from build123d import *

# Parameters (mm, degrees)
SKETCH1_R           = 2.5
SKETCH1_R_2         = 3.5
SKETCH1_R_3         = 1.5
SKETCH1_W           = 3
SKETCH1_H           = 10
BOSS_EXTRUDE3_DEPTH = 3


with BuildPart() as part:
    # Sketch1 → Boss-Extrude3 (new body)
    with BuildSketch(Plane(origin=(0, 0, 0), x_dir=(1, 0, 0), z_dir=(0, 1, 0))):
        with BuildLine():
            Line((36.277091695, 79.255784564), (46.277091695, 79.255784564))
            Line((46.277091695, 79.255784564), (46.277091695, 76.347710002))
            Line((46.277091695, 76.347710002), (71.277091695, 76.347710002))
            Line((71.277091695, 76.347710002), (71.277091695, 79.255784564))
            Line((71.277091695, 79.255784564), (82.277091695, 79.255784564))
            Line((82.277091695, 79.255784564), (82.277091695, -103.744215436))
            Line((82.277091695, -103.744215436), (71.277091695, -103.744215436))
            Line((71.277091695, -103.744215436), (71.277091695, -100.744215436))
            Line((71.277091695, -100.744215436), (46.277091695, -100.744215436))
            Line((46.277091695, -100.744215436), (46.277091695, -103.744215436))
            Line((46.277091695, -103.744215436), (36.277091695, -103.744215436))
            Line((36.277091695, -103.744215436), (36.277091695, 65.194662811))
            add(Edge.make_bspline(
                [(36.277091695, 73.316906316), (31.289085945, 73.316906316), (31.289085945, 69.255784564), (31.289085945, 65.194662811), (36.277091695, 65.194662811)],
                knots=[4.71238898, 4.71238898, 4.71238898, 6.283185307, 6.283185307, 7.853981634, 7.853981634, 7.853981634], degree=2, weights=[1, 0.707106781, 1, 0.707106781, 1]))
            Line((36.277091695, 73.316906316), (36.277091695, 79.255784564))
        make_face()
        with Locations(Location((35.277091695, 69.255784564, 0), (0, 0, 270))):
            Circle(SKETCH1_R, mode=Mode.SUBTRACT)
        with Locations(Location((62.277091695, 62.347710002, 0), (0, 0, 270))):
            Circle(SKETCH1_R_2, mode=Mode.SUBTRACT)
        with Locations(Location((62.277091695, 70.847710002, 0), (0, 0, 270))):
            Circle(SKETCH1_R_3, mode=Mode.SUBTRACT)
        with Locations(Location((62.277091695, 53.847710002, 0), (0, 0, 270))):
            Circle(SKETCH1_R_3, mode=Mode.SUBTRACT)
        with Locations(Location((62.277091695, -86.744215436, 0), (0, 0, 270))):
            Circle(SKETCH1_R_2, mode=Mode.SUBTRACT)
        with Locations(Location((62.277091695, -78.244215436, 0), (0, 0, 270))):
            Circle(SKETCH1_R_3, mode=Mode.SUBTRACT)
        with Locations(Location((62.277091695, -95.244215436, 0), (0, 0, 270))):
            Circle(SKETCH1_R_3, mode=Mode.SUBTRACT)
        with Locations((77.777091695, 43.827213135)):
            Rectangle(SKETCH1_W, SKETCH1_H, mode=Mode.SUBTRACT)
        with Locations((77.777091695, 66.255784564)):
            Rectangle(SKETCH1_W, SKETCH1_H, mode=Mode.SUBTRACT)
        with Locations((77.777091695, 21.398641707)):
            Rectangle(SKETCH1_W, SKETCH1_H, mode=Mode.SUBTRACT)
        with Locations((77.777091695, -1.029929722)):
            Rectangle(SKETCH1_W, SKETCH1_H, mode=Mode.SUBTRACT)
        with Locations((77.777091695, -23.458501151)):
            Rectangle(SKETCH1_W, SKETCH1_H, mode=Mode.SUBTRACT)
        with Locations((77.777091695, -45.887072579)):
            Rectangle(SKETCH1_W, SKETCH1_H, mode=Mode.SUBTRACT)
        with Locations((77.777091695, -68.315644008)):
            Rectangle(SKETCH1_W, SKETCH1_H, mode=Mode.SUBTRACT)
        with Locations((77.777091695, -90.744215436)):
            Rectangle(SKETCH1_W, SKETCH1_H, mode=Mode.SUBTRACT)
    extrude(amount=BOSS_EXTRUDE3_DEPTH)


solid = part.part
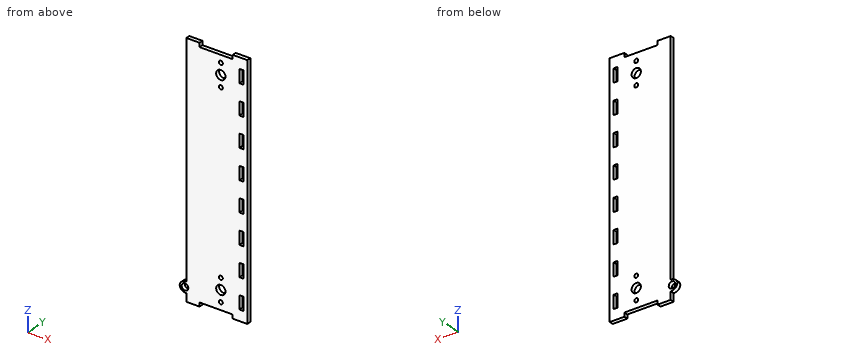
Verification items for the finished model (mm, model axes). Coordinates: 2 decimals unless noted, no trailing zeros. Loops run counter-clockwise (first coordinate to the right, second up) from the corner with the lowest first, then second, coordinate; pieces in that order, holes last. Notation, with made-up numbers: (17.25, -23.5) -> (56.25, -23.5) arc R11 ccw to (56.25, -17.5) -> close; hole circle Ø8 at (-26, 85.5). An arc over 180 degrees is marked (long way). Answer as a JSON object with one key per item and string values. Group by question number.
Item 1: Depth check by flat-ended pin: pin 1 (1.5 mm diameter, centred on y = 1.5, z = -76, fed in from -X); pin 2 (1.8 mm diameter, centred on x = 62.28, z = -53.85, fed in from +Y). Enter the tip coordinate at first touch or a pass-through.
Item 2: Sectioned sample at C-C on y = 1.9. State how many separate pieces and enclosed holes the cut face has, plus the area to 3 significant figures.
Item 3: Scan lines: probe 1 along X at (y, z) = (1, 19.5); probe 2 along Z at (x, y) = (59.5, 1.3); probe 3 along Z at (x, y) = (47.5, 1.4). Record each from-to range of solid material in increasing order.
Item 4: Sectioned sample at B-B on z = 56. Record the boundary of the cut face in (x, y), plus the area to 3 significant figures.
Item 5: Sectioned sample at A-A on z = 23.5. Record the boundary of the cut face in (x, y), plus the area to 3 significant figures.
Evaluation:
{
 "1": {"pin 1": "stops at x = 36.28", "pin 2": "passes through"},
 "2": {"separate pieces": "1", "enclosed holes": "15", "area": "7,940 mm²"},
 "3": {"probe 1": "x = 36.28 to 76.28, 79.28 to 82.28", "probe 2": "z = -76.35 to -64.48, -60.22 to 84.61, 88.87 to 100.74", "probe 3": "z = -76.35 to 100.74"},
 "4": {"outline": "(36.28, 0) -> (82.28, 0) -> (82.28, 3) -> (36.28, 3) -> close", "area": "138 mm²"},
 "5": {"outline": "(36.28, 0) -> (76.28, 0) -> (76.28, 3) -> (36.28, 3) -> close; (79.28, 0) -> (82.28, 0) -> (82.28, 3) -> (79.28, 3) -> close", "area": "129 mm²"}
}
